The listing builds one solid part. Answer for the finished solid, in the listing's coordinates (mm). Round coordinates to 2 decimals unless told otherwise and drop trailing zeros. Write each loop counter-clockwise with the first axis right and the second up, starting at its lowest first coordinate (ties: lowest second). Pieces come first, ordered by that corner, then holes. Notation, with made-up numbers: (-26, 37) - (8, 37) arc R31 cw to (8, 62) - close; hole circle Ø9 at (79, -32). An arc over 180 degrees is marked (long way). Return JSON: item names as keys, results as strings. Group by question number.
(1) Section B-B, the plane z = 40 is taken. Write down the section's boundary in (x, y), then the cut area to 3 significant figures.
(2) Determine the mould class of faces 1 (the cylindrical face through (-0.1, 12.3, -13.5)), 2 (the cylindrical face through (0.1, 12.3, 53.5)), 3 (the flat face through (0, 25, 20)), 4 (the cylindrical face through (-0.74, 12.32, 41.42)) for opening direction Z: +Z half, -Z half, draft (parallel to the pull), parting line (faces both ways), or undercut.
(3) Section C-C, the plane y = 11.5 is taken. Write down the section's boundary in (x, z), then the cut area to 3 significant figures.
(4) Section A-A, the plane x = 0 is taken. Write down the section's boundary in (y, z).
(5) This flat-tipped pin is pushed along its axis until it touches: pin 1 (1 mm diameter, centred on x = -2, y = 22, fed in from -Z). Where does it stop, or does it pass through?
(6) Find the intervals of material crossed by line 1 along Z through (x, y) = (0, 11.5); line 2 along Z through (x, y) = (0.5, 14.5); line 3 along Z through (x, y) = (2, 16.25), in increasing order. Write a range as [from, to].
(7) Section D-D, the plane z = -1 is taken. Write down the section's boundary in (x, y).
Autodesk Inventor part; units mm, degrees
ref_plane "YZ Plane" through (0, 0, 0) normal (1, 0, 0) x (0, 1, 0)
ref_plane "XZ Plane" through (0, 0, 0) normal (0, 1, 0) x (-1, 0, 0)
ref_plane "XY Plane" through (0, 0, 0) normal (0, 0, 1) x (1, 0, 0)
sketch "Sketch1" plane through (0, 0, 0) normal (0, 1, 0) x (-1, 0, 0)
  circle A0 centre (0, 0) radius 1.6
  line L0 (0, 0) -> (0, -10)
  circle A1 centre (0, -10) radius 1.6
  line L1 (0, 0) -> (0, 40)
  circle A2 centre (0, 40) radius 1.6
  line L2 (0, 40) -> (0, 50)
  circle A3 centre (0, 50) radius 1.6
  line L3 (0, 50) -> (0, -10) construction
  line L4 (-3.5, 50) -> (-3.5, -10)
  line L5 (3.5, -10) -> (3.5, 50)
  arc A4 (3.5, 50) -> (-3.5, 50) centre (0, 50) ccw
  arc A5 (-3.5, -10) -> (3.5, -10) centre (0, -10) ccw
  point P0 (0, 20)
  dimension "d0" = 3.2
  dimension "d1" = 10
  dimension "d2" = 3.2
  dimension "d3" = 40
  dimension "d4" = 3.2
  dimension "d5" = 10
  dimension "d6" = 3.2
  dimension "d7" = 7
extrude "Extrusion1" add sketch "Sketch1" along normal blind 25
properties part number "cover_wall_1"
Working result:
{
 "1": {"outline": "(-3.5, 0) - (-1.6, 0) - (-1.6, 25) - (-3.5, 25) - close; (1.6, 0) - (3.5, 0) - (3.5, 25) - (1.6, 25) - close", "area": "95.0 mm^2"},
 "2": {"face 1": "-Z half", "face 2": "+Z half", "face 3": "draft", "face 4": "undercut"},
 "3": {"outline": "(-3.5, -10) arc R3.5 ccw to (3.5, -10) - (3.5, 50) arc R3.5 ccw to (-3.5, 50) - close; hole circle Ø3.2 at (0, -10); hole circle Ø3.2 at (0, 0); hole circle Ø3.2 at (0, 40); hole circle Ø3.2 at (0, 50)", "area": "426 mm^2"},
 "4": {"outline": "(0, -13.5) - (25, -13.5) - (25, -11.6) - (0, -11.6) - close; (0, -8.4) - (25, -8.4) - (25, -1.6) - (0, -1.6) - close; (0, 1.6) - (25, 1.6) - (25, 38.4) - (0, 38.4) - close; (0, 41.6) - (25, 41.6) - (25, 48.4) - (0, 48.4) - close; (0, 51.6) - (25, 51.6) - (25, 53.5) - (0, 53.5) - close"},
 "5": {"pin 1": "stops at z = -13.16"},
 "6": {"line 1": "z = [-13.5, -11.6], [-8.4, -1.6], [1.6, 38.4], [41.6, 48.4], [51.6, 53.5]", "line 2": "z = [-13.46, -11.52], [-8.48, -1.52], [1.52, 38.48], [41.52, 48.48], [51.52, 53.46]", "line 3": "z = [-12.87, 52.87]"},
 "7": {"outline": "(-3.5, 0) - (-1.25, 0) - (-1.25, 25) - (-3.5, 25) - close; (1.25, 0) - (3.5, 0) - (3.5, 25) - (1.25, 25) - close"}
}
